The listing builds one solid part. Answer for the finished solid, in the listing's coordinates (mm). A direction names the side the tool comes from. Coordinates: 2 decimals unless noted, no trailing zeros. Write each loop counter-clockwise with the first axis right and the second up, starting at its lowest first coordinate (ties: lowest second). Pieces come first, ordered by that corner, then holes. Notation, with made-up numbers: M 22.5,-36 L 34.5,-36 A13 cw 34.5,-32 Z; hole C -33.5,71 d8. An arc over 180 degrees is marked long. Put each result on its own line as item: value. Start each with the question number.
```python
from build123d import *

# Parameters (mm, degrees)
SKETCH1_W           = 9.525
SKETCH1_H           = 19.05
SKETCH1_W_2         = 3.175
BOSS_EXTRUDE1_DEPTH = 3.175
BOSS_EXTRUDE2_START = 3.175
SKETCH1_3_W         = 3.175
SKETCH1_3_H         = 19.05
BOSS_EXTRUDE2_DEPTH = 12.7
SKETCH2_R           = 2
CUT_EXTRUDE1_DEPTH  = 21.819867315


with BuildPart() as part:
    # Sketch1 → Boss-Extrude1 (new body)
    with BuildSketch(Plane(origin=(0, 0, 0), x_dir=(1, 0, 0), z_dir=(0, 1, 0))):
        with Locations((1.5875, 0)):
            Rectangle(SKETCH1_W, SKETCH1_H)
        with Locations((-4.7625, 0)):
            Rectangle(SKETCH1_W_2, SKETCH1_H)
    extrude(amount=BOSS_EXTRUDE1_DEPTH)

    # Sketch1<3> → Boss-Extrude2 (add)
    with BuildSketch(Plane(origin=(0, 0, 0), x_dir=(1, 0, 0), z_dir=(0, 1, 0)).offset(BOSS_EXTRUDE2_START)):
        with Locations((-4.7625, 0)):
            Rectangle(SKETCH1_3_W, SKETCH1_3_H)
    extrude(amount=BOSS_EXTRUDE2_DEPTH)

    # Sketch2 → Cut-Extrude1 (cut, through all)
    with BuildSketch(Plane(origin=(-3.175, 0, 0), x_dir=(0, 0, -1), z_dir=(1, 0, 0))):
        with Locations((0, 12.7)):
            Circle(SKETCH2_R)
    extrude(amount=-CUT_EXTRUDE1_DEPTH, mode=Mode.SUBTRACT)


solid = part.part
```
1) A cutting plane is placed at D-D on x = 1. Write down the section's boundary in (y, z) (3 decimals), then the cut area to 3 significant figures.
2) A cutting plane is placed at A-A on y = 12.7. Write down the section's boundary in (x, z) (3 decimals), then the cut area to 3 significant figures.
3) Straight lines are drawn through the part: probe 1 along Y at (x, z) = (-5.45, 0) (3 decimals); probe 2 along X at (y, z) = (4.75, 8.75) (3 decimals); probe 3 along Y at (x, z) = (1.5, -8) (3 decimals). For each, find the intervals that lie inside material, in ascending order.
4) Given pin 1 Ø3.5 at (y, z) = (12.7, 0) entering from -X; pin 2 Ø5 at (x, z) = (0, -4) entering from +Y (3 decimals); pin 3 Ø6.5 at (y, z) = (7.5, 0) entering from +X (3 decimals), each flat-ended and moving along its own axis, determine where each tip first touches the part or whether it passes through.
5) A cutting plane is placed at C-C on z = 7.5. Write down the section's boundary in (x, y) (3 decimals), then the cut area to 3 significant figures.
6) A cutting plane is placed at B-B on z = 0. Write down the section's boundary in (x, y) (3 decimals).
7) For faces 1 (the face through (-4, 4, 9.525)), 2 (the face through (-3.175, 9, 0)), determine the directions among +Z, -Z, +X, -X, +Y, -Y from which every point of the face is accessible in a straight line to the end or side of a thin tool.
8) Determine the mould class of faces 3 (the face through (-4, 4, -9.525)), 4 (the face through (0, 0, 0)), 5 (the face through (-4.74, 10.748, 0.434)), 6 (the face through (2, 3.175, 0)) for opening direction Y: +Y half, -Y half, draft (parallel to the pull), parting line (faces both ways), or undercut.
Answers follow:
1. outline: M 0,-9.525 L 3.175,-9.525 L 3.175,9.525 L 0,9.525 Z
1. area: 60.5 mm²
2. outline: M -6.35,-9.525 L -3.175,-9.525 L -3.175,-2 L -6.35,-2 Z; M -6.35,2 L -3.175,2 L -3.175,9.525 L -6.35,9.525 Z
2. area: 47.8 mm²
3. probe 1: y = 0 to 10.7, 14.7 to 15.875
3. probe 2: x = -6.35 to -3.175
3. probe 3: y = 0 to 3.175
4. pin 1: passes through
4. pin 2: stops at y = 3.175
4. pin 3: stops at x = -3.175
5. outline: M -6.35,0 L 6.35,0 L 6.35,3.175 L -3.175,3.175 L -3.175,15.875 L -6.35,15.875 Z
5. area: 80.6 mm²
6. outline: M -6.35,0 L 6.35,0 L 6.35,3.175 L -3.175,3.175 L -3.175,10.7 L -6.35,10.7 Z; M -6.35,14.7 L -3.175,14.7 L -3.175,15.875 L -6.35,15.875 Z
7. face 1: +Z, +X, -X, +Y, -Y
7. face 2: +Z, -Z, +X, +Y
8. face 3: draft
8. face 4: -Y half
8. face 5: undercut
8. face 6: +Y half
